Autodesk Inventor part; units mm, degrees
ref_plane "YZ Plane" through (0, 0, 0) normal (1, 0, 0) x (0, 1, 0)
ref_plane "XZ Plane" through (0, 0, 0) normal (0, 1, 0) x (-1, 0, 0)
ref_plane "XY Plane" through (0, 0, 0) normal (0, 0, 1) x (1, 0, 0)
sketch "草图1" plane through (0, 0, 0) normal (0, 0, 1) x (1, 0, 0)
  arc A0 (28.5, 0) -> (-28.5, 0) centre (0, 0) ccw
  line L0 (-50, 0) -> (50, 0)
  line L1 (50, 0) -> (50, 5)
  line L2 (50, 5) -> (-50, 5)
  line L3 (-50, 5) -> (-50, 0)
  dimension "d0" = 57
  dimension "d1" = 100
  dimension "d2" = 5
extrude "拉伸1" add sketch "草图1" along normal blind 30
sketch "草图2" plane through (0, 0, 30) normal (0, 0, 1) x (1, 0, 0)
  circle A0 centre (0, 0) radius 18.5
  dimension "d5" = 37
extrude "拉伸2" cut sketch "草图2" against normal blind 9
sketch "草图3" plane through (0, 0, 21) normal (0, 0, 1) x (1, 0, 0)
  circle A0 centre (0, 0) radius 14
  dimension "d8" = 28
extrude "拉伸3" cut sketch "草图3" against normal blind 5
sketch "草图4" plane through (0, 0, 16) normal (0, 0, 1) x (1, 0, 0)
  circle A0 centre (0, 0) radius 10
  dimension "d11" = 20
extrude "拉伸4" cut sketch "草图4" against normal through all
fillet "圆角1" radius 4 2 edges at (28.058, 5, 15) (-28.058, 5, 15)
sketch "草图5" plane through (50, 5, 30) normal (0, 1, 0) x (1, 0, 0)
  circle A0 centre (-7, 23) radius 2.5
  circle A1 centre (-7, 7) radius 2.5
  circle A2 centre (-93, 7) radius 2.5
  circle A3 centre (-93, 23) radius 2.5
  line L0 (-81.229, 30) -> (-100, 30)
  line L1 (-100, 30) -> (-100, 0)
  line L2 (-81.229, 0) -> (-100, 0)
  line L3 (0, 30) -> (-18.771, 30)
  line L4 (0, 30) -> (0, 0)
  line L5 (0, 0) -> (-18.771, 0)
  point P0 (-50, 30)
  dimension "d15" = 5
  dimension "d16" = 5
  dimension "d17" = 5
  dimension "d18" = 5
  dimension "d19" = 7
  dimension "d20" = 7
  dimension "d21" = 7
  dimension "d22" = 7
  dimension "d23" = 7
  dimension "d24" = 7
  dimension "d25" = 7
  dimension "d26" = 7
extrude "拉伸5" cut sketch "草图5" against normal through all
properties part number "砂轮架带动曲轴固定盖"
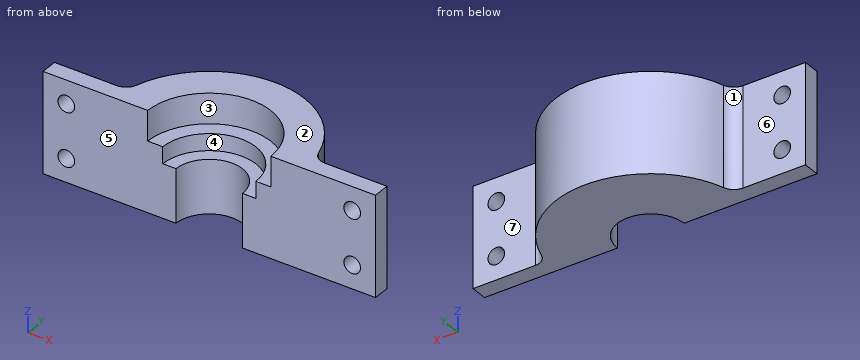
Verification items for the finished model (mm, model axes). Face numbers are marked on the shaded views. A direction names the side the tool comes from. Round coordinates to 2 decimals unless told otherwise and drop trailing zeros. Loops run counter-clockwise (first coordinate to the right, second up) from the corner with the lowest first, then second, coordinate; pieces in that order, holes last. Notation, with made-up numbers: (29, -12) -> (46, -12) arc R37 ccw to (46, 26) -> close; hole circle Ø7 at (-23.75, 57). An arc over 180 degrees is marked (long way). Answer as a JSON object with one key per item and string values.
Q1. Section check C-C (x = 0). Record the boundary of the cut face in (y, z).
Data:
{"outline": "(10, 0) -> (28.5, 0) -> (28.5, 30) -> (18.5, 30) -> (18.5, 21) -> (14, 21) -> (14, 16) -> (10, 16) -> close"}
Q2. Section check D-D (z = 13). Record the boundary of the cut face in (x, y).
Data:
{"outline": "(-50, 0) -> (-10, 0) arc R10 cw to (10, 0) -> (50, 0) -> (50, 5) -> (31.23, 5) arc R4 cw to (27.39, 7.89) arc R28.5 ccw to (-27.39, 7.89) arc R4 cw to (-31.23, 5) -> (-50, 5) -> close"}
Q3. Scan lines: line 1 (Z direction, x = -43, y = 3.15); line 2 (X direction, y = 1.6, z = 23); line 3 (X direction, y = 1.2, z = 7). Record each from-to range of solid material in increasing order. Write a range as from..to.
Data:
{"line 1": "z = 0..4.5, 9.5..20.5, 25.5..30", "line 2": "x = -50..-45.5, -40.5..-18.43, 18.43..40.5, 45.5..50", "line 3": "x = -50..-45.5, -40.5..-9.93, 9.93..40.5, 45.5..50"}
Q4. Go/stop test with flat-tipped pins: P1, Ø5, axis at x = 36, z = 12.5, coming from the +Y side; P2, Ø12, axis at y = 23, z = 25.5, coming from the +X side; P3, Ø3, axis at x = 43, z = 23, coming from the +Y side; P4, Ø5.5, axis at x = 8.5, y = 11, coming from the +Z side. Record where each tip stops, or that it passes through.
Data:
{"P1": "stops at y = 5", "P2": "stops at x = 22.87", "P3": "passes through", "P4": "stops at z = 21"}
Q5. Draft check along X on the marked faces 1, 2, 3 and 4. Enter one of: pulls with the +X half, pulls with the -X half, needs draft (parallel to the pull), parting line crosses it, or undercut.
Data:
{"face 1": "pulls with the -X half", "face 2": "needs draft", "face 3": "undercut", "face 4": "undercut"}
Q6. Access from +Z, -Z, +X, -X, +Y, -Y to the whole of each face (thin tool, end or side, straight path). Record for the marked faces 5, 6 and 7.
Data:
{"face 5": "+Z, -Z, +X, -X, -Y", "face 6": "+Z, -Z, -X, +Y", "face 7": "+Z, -Z, +X, +Y"}
Q7. Section check A-A (z = 7). Record the boundary of the cut face in (x, y), then the cut area to 3 significant figures.
Data:
{"outline": "(-50, 0) -> (-45.5, 0) -> (-45.5, 5) -> (-50, 5) -> close; (-40.5, 0) -> (-10, 0) arc R10 cw to (10, 0) -> (40.5, 0) -> (40.5, 5) -> (31.23, 5) arc R4 cw to (27.39, 7.89) arc R28.5 ccw to (-27.39, 7.89) arc R4 cw to (-31.23, 5) -> (-40.5, 5) -> close; (45.5, 0) -> (50, 0) -> (50, 5) -> (45.5, 5) -> close", "area": "1,290 mm2"}
Q8. Section check B-B (x = -43). Record the boundary of the cut face in (y, z), then the cut area to 3 significant figures.
Data:
{"outline": "(0, 0) -> (5, 0) -> (5, 4.5) -> (0, 4.5) -> close; (0, 9.5) -> (5, 9.5) -> (5, 20.5) -> (0, 20.5) -> close; (0, 25.5) -> (5, 25.5) -> (5, 30) -> (0, 30) -> close", "area": "100 mm2"}
